from build123d import *

# Parameters (mm, degrees)
F0_W     = 63.5
F0_H     = 63.5
F0_W_2   = 57.15
F0_H_2   = 57.15
F0_W_3   = 50.8
F0_H_3   = 50.8
F1_DEPTH = 16.9333333333
F0_W_4   = 69.85
F0_H_4   = 69.85
F2_DEPTH = 12.7
F0_W_5   = 75.946
F0_H_5   = 75.946
F3_DEPTH = 8.4666666667
F0_W_6   = 76.2
F0_H_6   = 76.2
F4_DEPTH = 4.2333333333
F5_DEPTH = 6.35


with BuildPart() as f1:
    # F0 (on Top) → F1 (new body)
    with BuildSketch(Plane.XY):
        Rectangle(F0_W, F0_H)
        Rectangle(F0_W_2, F0_H_2, mode=Mode.SUBTRACT)
        Rectangle(F0_W_2, F0_H_2)
        Rectangle(F0_W_3, F0_H_3, mode=Mode.SUBTRACT)
        Rectangle(F0_W_3, F0_H_3)
    extrude(amount=F1_DEPTH)

    # F0 (on Top) → F2 (join)
    with BuildSketch(Plane.XY):
        Rectangle(F0_W_4, F0_H_4)
        Rectangle(F0_W, F0_H, mode=Mode.SUBTRACT)
    extrude(amount=F2_DEPTH)

    # F0 (on Top) → F3 (join)
    with BuildSketch(Plane.XY):
        Rectangle(F0_W_5, F0_H_5)
        Rectangle(F0_W_4, F0_H_4, mode=Mode.SUBTRACT)
    extrude(amount=F3_DEPTH)

    # F0 (on Top) → F4 (join)
    with BuildSketch(Plane.XY):
        Rectangle(F0_W_6, F0_H_6)
        Rectangle(F0_W_5, F0_H_5, mode=Mode.SUBTRACT)
    extrude(amount=F4_DEPTH)

    # F5 (add): a face of the model
    f5_faces = [f1.faces().sort_by_distance(p)[0] for p in [
        (0, 0, 0),
    ]]
    extrude(f5_faces, amount=F5_DEPTH)


solid = f1.part
Input: part model. Units: mm. Frame: model coordinates. A direction names the side the tool comes from. Give positions to 0.01 mm unless a question says otherwise; leave off trailing zeros. Order: outer loops, then holes, each group sorted by start corner. A loop starts at its lowest first (then second) coordinate and runs counter-clockwise, first axis right, second up.
Q1. Ray query, probe 1 along Y at (x, z) = (-19.5, 9.5) (3 decimals); probe 2 along Y at (x, z) = (15.5, 13.5); probe 3 along Z at (x, y) = (32.5, -28). Return the intervals inside material, ascending.
Checked values:
probe 1: y = -34.925 to 34.925
probe 2: y = -31.75 to 31.75
probe 3: z = -6.35 to 12.7
Q2. Section C-C on z = 9.5. Output: boundary loops of the cut face in (x, y) (3 decimals), and give its area (3 significant figures).
Checked values:
outline: (-34.925, -34.925) - (34.925, -34.925) - (34.925, 34.925) - (-34.925, 34.925) - close
area: 4,880 mm2
Q3. Section A-A on y = 33.5. Output: boundary loops of the cut face in (x, z) (3 decimals).
Checked values:
outline: (-38.1, -6.35) - (38.1, -6.35) - (38.1, 4.233) - (37.973, 4.233) - (37.973, 8.467) - (34.925, 8.467) - (34.925, 12.7) - (-34.925, 12.7) - (-34.925, 8.467) - (-37.973, 8.467) - (-37.973, 4.233) - (-38.1, 4.233) - close
Q4. Set-up query: faces 1 (the flat face through (0, -34.925, 11)), 2 (the flat face through (0, 31.75, 15)), 3 (the flat face through (31.75, 0, 15)), 4 (the flat face through (-37.973, -1, 6)). Return all of +Z, -Z, +X, -X, +Y, -Y with unobstructed straight access to the full face (end or side cutting, diameter ignored); none if empty.
Checked values:
face 1: +Z, +X, -X, -Y
face 2: +Z, +X, -X, +Y
face 3: +Z, +X, +Y, -Y
face 4: +Z, -X, +Y, -Y
Q5. Section B-B on x = 20. Output: boundary loops of the cut face in (y, z) (3 decimals).
Checked values:
outline: (-38.1, -6.35) - (38.1, -6.35) - (38.1, 4.233) - (37.973, 4.233) - (37.973, 8.467) - (34.925, 8.467) - (34.925, 12.7) - (31.75, 12.7) - (31.75, 16.933) - (-31.75, 16.933) - (-31.75, 12.7) - (-34.925, 12.7) - (-34.925, 8.467) - (-37.973, 8.467) - (-37.973, 4.233) - (-38.1, 4.233) - close
Q6. Contact query for flat-ended pins moving along their axis: pin 1 Ø4.5 at (x, z) = (-12.5, 11.5) entering from +Y (3 decimals); pin 2 Ø3.5 at (x, z) = (11, 14.5) entering from -Y; pin 3 Ø3.5 at (y, z) = (-2, 16) entering from -X. Output: stop coordinate, or through.
Checked values:
pin 1: stops at y = 34.925
pin 2: stops at y = -31.75
pin 3: stops at x = -31.75
